Work out the finished part from the listing and answer in its coordinate system (mm). Coordinates: 2 decimals unless noted, no trailing zeros. Order: outer loops, then holes, each group sorted by start corner. A loop starts at its lowest first (then second) coordinate and runs counter-clockwise, first axis right, second up. Notation, with made-up numbers: (35, 2.5) -> (50, 2.5) arc R24 ccw to (50, 30.5) -> close; hole circle Ø4 at (-23.75, 18.5). An arc over 180 degrees is marked (long way). Answer as CSV lines item,"result". Start each with the question number.
Item 1: Section D-D (y = -18) is taken. Write down the section's boundary in (x, z), then the cut area to 3 significant figures.
Item 2: Section A-A (x = 16) is taken. Write down the section's boundary in (y, z), then the cut area to 3 significant figures.
Item 3: Straight lines are drawn through the part: L1, parallel to Y at x = 14.5, z = -22.5; L2, parallel to Z at x = -13.5, y = -2.5; L3, parallel to Z at x = 30.5, y = 9. For each, find the intervals that lie inside material, in ascending order.
Item 4: Section C-C (y = 28.5) is taken. Write down the section's boundary in (x, z).
Item 5: Section B-B (z = -3.5) is taken. Write down the section's boundary in (x, y), then the cut area to 3 significant figures.
Item 6: Each of these flat-tipped pins is pushed along its axis until it touches: pin 1 Ø2 at (x, y) = (35.5, 35) entering from -Z; pin 2 Ø5 at (x, y) = (-6.5, 38.5) entering from +Z; pin 3 Ø6 at (x, y) = (23.5, 33.5) entering from -Z. Where does it stop, or does it pass through?
```python
from build123d import *

# Parameters (mm, degrees)
F0_W     = 50.0006489456
F0_H     = 50.0006489456
F1_DEPTH = 50
F3_ANGLE = 45
F5_ANGLE = 45


with BuildPart() as f1:
    # F0 (on Top) → F1 (new body)
    with BuildSketch(Plane.XY):
        Rectangle(F0_W, F0_H)
    extrude(amount=F1_DEPTH)


with BuildPart() as f1_1:
    # F2: moved
    add(f1.part.moved(Location((0, 0, -25))))


with BuildPart() as f1_2:
    # F3: moved
    add(f1_1.part.rotate(Axis((25.0003244728, -25.0003244728, 0), (0, 0, -1)), F3_ANGLE))


with BuildPart() as f1_3:
    # F5: moved
    add(f1_2.part.rotate(Axis((0, 20.7308493555, 0), (0, 1, 0)), F5_ANGLE))


solid = f1_3.part
```
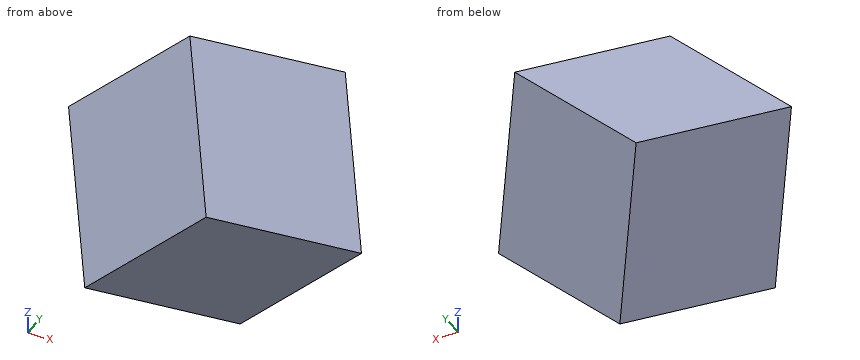
Checked values:
1,outline,"(-4.95, -30.41) -> (4.95, -40.31) -> (40.31, -4.95) -> (30.41, 4.95) -> close"
1,area,"700 mm^2"
2,outline,"(-25, -19.36) -> (-2.37, -51.36) -> (23.08, -51.36) -> (45.71, -19.36) -> (18.34, 19.36) -> (2.37, 19.36) -> close"
2,area,"3,220 mm^2"
3,L1,"y = -23.84 to 44.55"
3,L2,"z = -21.86 to -17.04"
3,L3,"z = -52.94 to 4.86"
4,outline,"(-12.17, -23.19) -> (12.17, -47.53) -> (47.53, -12.17) -> (23.19, 12.17) -> close"
5,outline,"(-18.14, 10.36) -> (31.86, -25) -> (38.86, -20.05) -> (38.86, 40.76) -> (31.86, 45.71) -> close"
5,area,"2,230 mm^2"
6,pin 1,"stops at z = -16.74"
6,pin 2,"stops at z = -27.33"
6,pin 3,"stops at z = -34.32"
